For this review, use the dimensioned drawing (mm, ordinates from the lowest corner) and the shaded views. A direction names the side the tool comes from. Give positions to 0.01 mm unless a question says otherwise; leave off trailing zeros. Order: outer loops, then holes, each group sorted by start corner. A loop starts at its lowest first (then second) coordinate and runs counter-clockwise, first axis right, second up.
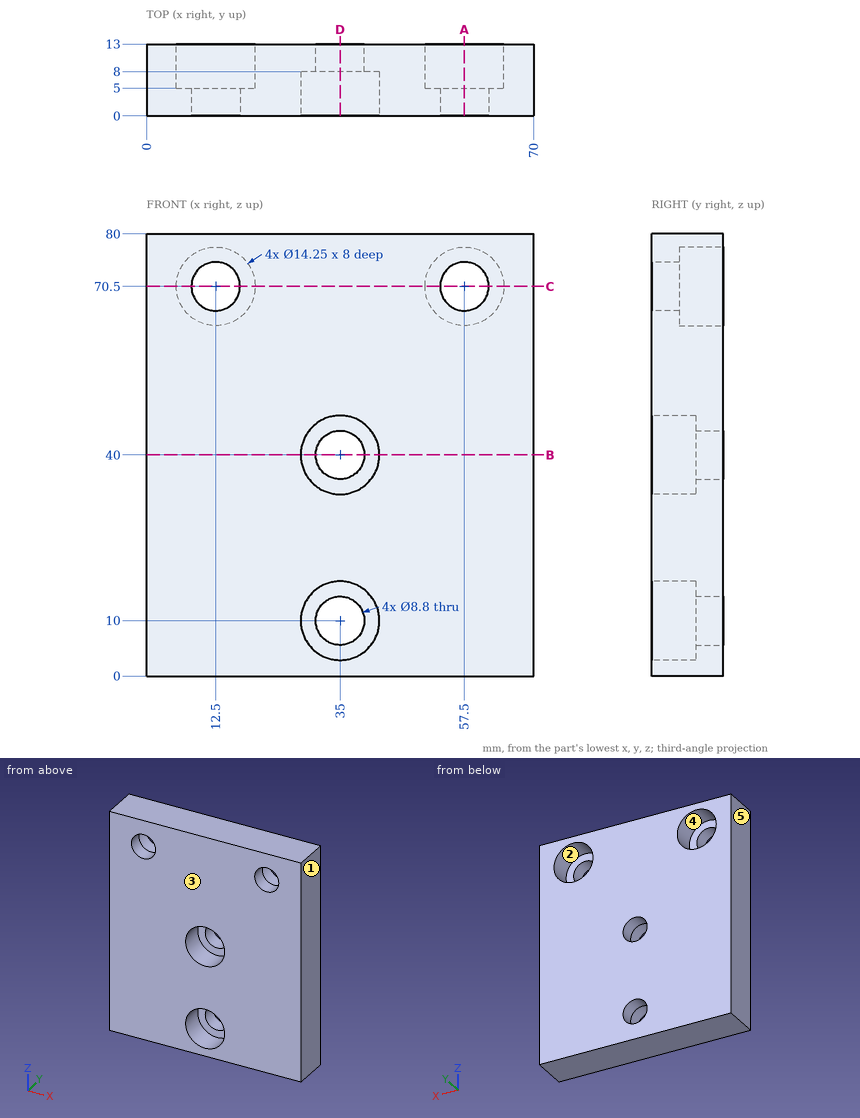
1. Take a section at B-B (z = 40). State the section outline as (x, y) points (3 decimals), then the cut area to 3 significant figures.
Recorded:
outline: (0, 0) - (27.875, 0) - (27.875, 8) - (30.6, 8) - (30.6, 13) - (0, 13) - close; (39.4, 8) - (42.125, 8) - (42.125, 0) - (70, 0) - (70, 13) - (39.4, 13) - close
area: 752 mm2
2. Take a section at D-D (x = 35). State the section outline as (y, z) points (3 decimals), then the cut area to 3 significant figures.
Recorded:
outline: (0, 0) - (13, 0) - (13, 5.6) - (8, 5.6) - (8, 2.875) - (0, 2.875) - close; (0, 17.125) - (8, 17.125) - (8, 14.4) - (13, 14.4) - (13, 35.6) - (8, 35.6) - (8, 32.875) - (0, 32.875) - close; (0, 47.125) - (8, 47.125) - (8, 44.4) - (13, 44.4) - (13, 80) - (0, 80) - close
area: 724 mm2
3. Take a section at A-A (x = 57.5). State the section outline as (y, z) points (3 decimals).
Recorded:
outline: (0, 0) - (13, 0) - (13, 63.375) - (5, 63.375) - (5, 66.1) - (0, 66.1) - close; (0, 74.9) - (5, 74.9) - (5, 77.625) - (13, 77.625) - (13, 80) - (0, 80) - close
4. For line 1 along Z through (x, y) = (35, 9.85); line 2 along Z through (x, y) = (35, 3) (3 decimals); line 3 along Z through (x, y) = (57.5, 11) (3 decimals), list the stretches that pass through material, from the lowest coordinate up.
Recorded:
line 1: z = 0 to 5.6, 14.4 to 35.6, 44.4 to 80
line 2: z = 0 to 2.875, 17.125 to 32.875, 47.125 to 80
line 3: z = 0 to 63.375, 77.625 to 80
5. Draft analysis for pull direction X (two halves, no side actions). For the marked faces 1, 2 and 3, state which applies: pulls with the +X half, pulls with the -X half, needs draft (parallel to the pull), parting line crosses it, or undercut.
Recorded:
face 1: pulls with the +X half
face 2: undercut
face 3: needs draft
6. Machinability: for the marked faces 4 and 5, which of the approach directions +Z, -Z, +X, -X, +Y, -Y give a long, thin tool a straight path to every point of the face, cutting with its end or side? Answer none if there is none.
Recorded:
face 4: +Y
face 5: +Z, -Z, -X, +Y, -Y
7. Take a section at C-C (z = 70.5). State the section outline as (x, y) points (3 decimals), then the cut area to 3 significant figures.
Recorded:
outline: (0, 0) - (8.1, 0) - (8.1, 5) - (5.375, 5) - (5.375, 13) - (0, 13) - close; (16.9, 0) - (53.1, 0) - (53.1, 5) - (50.375, 5) - (50.375, 13) - (19.625, 13) - (19.625, 5) - (16.9, 5) - close; (61.9, 0) - (70, 0) - (70, 13) - (64.625, 13) - (64.625, 5) - (61.9, 5) - close
area: 594 mm2
8. For pin 1 (7 mm diameter, centred on x = 35, z = 40, fed in from +Y); pin 2 (7 mm diameter, centred on x = 37, z = 7.5, fed in from -Y), all flat-tipped, find the tip position at first contact; note any pin that passes through.
Recorded:
pin 1: passes through
pin 2: stops at y = 8
